Could you check a few things on this model? Use its own coordinates, in mm. Face numbers are marked on the shaded views. A direction names the side the tool comes from. Round coordinates to 2 decimals unless told otherwise and drop trailing zeros. Loops run counter-clockwise (first coordinate to the right, second up) from the corner with the lowest first, then second, coordinate; pieces in that order, holes last. Notation, with made-up numbers: M 25.25,78.25 L 39.25,78.25 A16 cw 39.25,87.25 Z; hole C -11.5,66 d2. An arc over 180 degrees is marked long. Return JSON: item names as keys, results as strings. Group by question number.
```python
from build123d import *

# Parameters (mm, degrees)
SKETCH1_W           = 12.9
SKETCH1_H           = 5.8
BOSS_EXTRUDE1_DEPTH = 6.2
SKETCH2_W           = 0.389977013
SKETCH2_H           = 2.515896803
BOSS_EXTRUDE2_DEPTH = 1
SKETCH3_W           = 0.417854015
SKETCH3_H           = 2.825804308
SKETCH3_W_2         = 0.316823763
SKETCH3_W_3         = 0.356926389
BOSS_EXTRUDE3_DEPTH = 5


with BuildPart() as part:
    # Sketch1 → Boss-Extrude1 (new body)
    with BuildSketch(Plane(origin=(0, 0, 0), x_dir=(1, 0, 0), z_dir=(0, 1, 0))):
        with Locations((6.45, -2.9)):
            Rectangle(SKETCH1_W, SKETCH1_H)
    extrude(amount=BOSS_EXTRUDE1_DEPTH)

    # Sketch2 → Boss-Extrude2 (add)
    with BuildSketch(Plane(origin=(0, 6.2, 0), x_dir=(1, 0, 0), z_dir=(0, 1, 0))):
        with Locations((1.343594609, -2.794175743)):
            Rectangle(SKETCH2_W, SKETCH2_H)
    extrude(amount=BOSS_EXTRUDE2_DEPTH)

    # Sketch3 → Boss-Extrude3 (add)
    with BuildSketch(Plane(origin=(0, 0, 0), x_dir=(-1, 0, 0), z_dir=(0, -1, 0))):
        with Locations((-1.673057287, -3.048690626)):
            Rectangle(SKETCH3_W, SKETCH3_H)
        with Locations((-6.194757306, -3.048690626)):
            Rectangle(SKETCH3_W_2, SKETCH3_H)
        with Locations((-10.065176498, -3.048690626)):
            Rectangle(SKETCH3_W_3, SKETCH3_H)
    extrude(amount=BOSS_EXTRUDE3_DEPTH)


solid = part.part
```
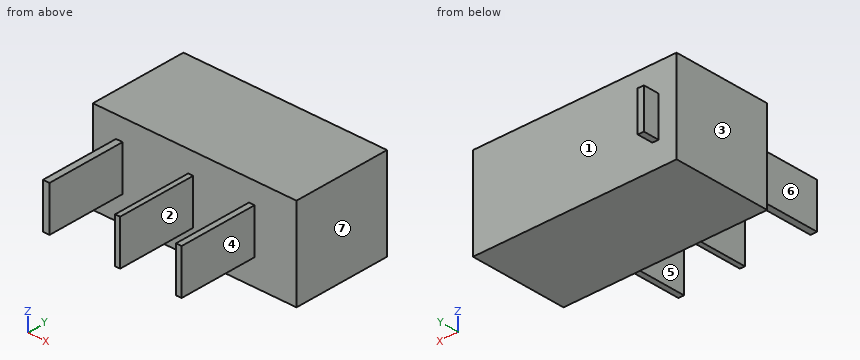
1. If we section it at D-D, the plane z = 5: Please give me the cut outline in (x, y).
2. If we section it at C-C, the plane x = 4: Please give me the cut outline in (y, z).
3. We'd pull the mould along X, two halves only. Please class the marked faces 1, 2 and 3: +X half, -X half, draft (parallel to the pull), parting line (faces both ways), or undercut.
4. I need wall thicknesses on probe 1 along X at (y, z) = (-1, 2.5); probe 2 along Y at (x, z) = (6.25, 5.35). Which ranges of each line are inside material? Lowest first, please.
5. If we section it at B-B, the plane z = 1.9: Please give me the cut outline in (x, y), then the cut area to 3 significant figures.
6. I'm going to push flat-ended pins straight in: pin 1 Ø1.4 at (y, z) = (-2.5, 2.5) entering from -X; pin 2 Ø3 at (x, z) = (6, 4) entering from +Y; pin 3 Ø2.5 at (y, z) = (-3, 2.5) entering from +X. Where does each tip first touch, or does it pass through?
7. If we section it at A-A, the plane y = -0.5: Please give me the cut outline in (x, z).
8. On a 3-axis mill with a long thin cutter (end or side, diameter ignored), from which of +Z, -Z, +X, -X, +Y, -Y can I reach the whole of each face in a straight line? I mean the marked faces 4, 5, 6 and 7. Say none if no direction works.
Geometry results:
{
 "1": {"outline": "M 0,0 L 12.9,0 L 12.9,6.2 L 0,6.2 Z"},
 "2": {"outline": "M 0,0 L 6.2,0 L 6.2,5.8 L 0,5.8 Z"},
 "3": {"face 1": "draft", "face 2": "undercut", "face 3": "-X half"},
 "4": {"probe 1": "1.46 to 1.88, 6.04 to 6.35, 9.89 to 10.24", "probe 2": "0 to 6.2"},
 "5": {"outline": "M 0,0 L 1.46,0 L 1.46,-5 L 1.88,-5 L 1.88,0 L 6.04,0 L 6.04,-5 L 6.35,-5 L 6.35,0 L 9.89,0 L 9.89,-5 L 10.24,-5 L 10.24,0 L 12.9,0 L 12.9,6.2 L 1.54,6.2 L 1.54,7.2 L 1.15,7.2 L 1.15,6.2 L 0,6.2 Z", "area": "85.8 mm^2"},
 "6": {"pin 1": "x = 1.46", "pin 2": "y = 6.2", "pin 3": "x = 10.24"},
 "7": {"outline": "M 1.46,1.64 L 1.88,1.64 L 1.88,4.46 L 1.46,4.46 Z; M 6.04,1.64 L 6.35,1.64 L 6.35,4.46 L 6.04,4.46 Z; M 9.89,1.64 L 10.24,1.64 L 10.24,4.46 L 9.89,4.46 Z"},
 "8": {"face 4": "+Z, -Z, +X, -Y", "face 5": "+Z, -Z, -Y", "face 6": "+Z, -Z, -X, -Y", "face 7": "+Z, -Z, +X, +Y, -Y"}
}
